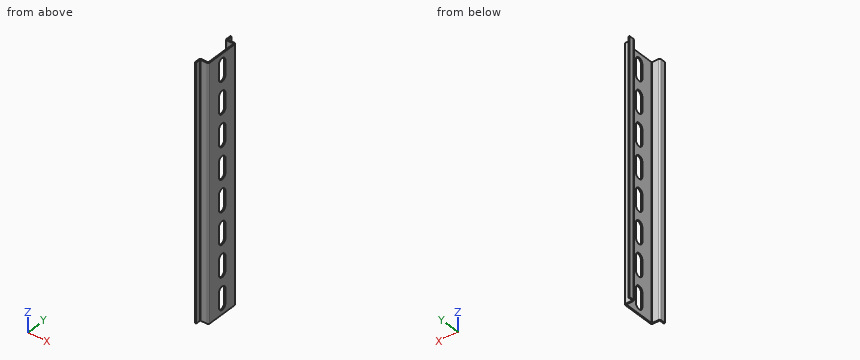
```python
from build123d import *

# Parameters (mm, degrees)
EXTRUDE_THIN1_DEPTH = 200.025
CUT_EXTRUDE1_START  = -8.5
CUT_EXTRUDE1_DEPTH  = 9.5
LPATTERN1_COUNT     = 32
LPATTERN1_PITCH     = 25
FILLET1_R           = 0.25
FILLET2_R           = 1.25


with BuildPart() as part:
    # Sketch3 → Extrude-Thin1 (new body)
    with BuildSketch(Plane.XY):
        Polygon((-6.5, 17.5), (-6.5, 13.5), (0, 13.5), (0, -13.5), (-6.5, -13.5), (-6.5, -17.5), (-7.5, -17.5), (-7.5, -12.5), (-1, -12.5), (-1, 12.5), (-7.5, 12.5), (-7.5, 17.5), align=None)
    extrude(amount=EXTRUDE_THIN1_DEPTH)

    # Sketch4 → Cut-Extrude1 (cut)
    with BuildSketch(Plane(origin=(0, 0, 0), x_dir=(0, 0, -1), z_dir=(1, 0, 0)).offset(CUT_EXTRUDE1_START)):
        with BuildLine():
            Line((-6.65, -3.15), (-18.35, -3.15))
            ThreePointArc((-18.35, -3.15), (-21.5, 0), (-18.35, 3.15))
            Line((-18.35, 3.15), (-6.65, 3.15))
            ThreePointArc((-6.65, 3.15), (-3.5, 0), (-6.65, -3.15))
        make_face()
    cut_extrude1 = extrude(amount=CUT_EXTRUDE1_DEPTH, mode=Mode.SUBTRACT)

    # LPattern1: Cut-Extrude1 ×32
    with Locations(*[(0, 0, i * LPATTERN1_PITCH) for i in range(1, LPATTERN1_COUNT)]):
        add(cut_extrude1, mode=Mode.SUBTRACT)

    # Fillet1
    fillet1_edges = [part.edges().sort_by_distance(p)[0] for p in [
        (-6.5, 13.5, 100.0125),
        (-6.5, -13.5, 100.0125),
        (-1, -12.5, 100.0125),
        (-1, 12.5, 100.0125),
    ]]
    fillet(fillet1_edges, radius=FILLET1_R)

    # Fillet2
    fillet2_edges = [part.edges().sort_by_distance(p)[0] for p in [
        (0, 13.5, 100.0125),
        (0, -13.5, 100.0125),
        (-7.5, -12.5, 100.0125),
        (-7.5, 12.5, 100.0125),
    ]]
    fillet(fillet2_edges, radius=FILLET2_R)


solid = part.part
```
Geometry check sheet. Reference: the model listing, model coordinates, mm. Round coordinates to 2 decimals unless told otherwise and drop trailing zeros. Order: outer loops, then holes, each group sorted by start corner. A loop starts at its lowest first (then second) coordinate and runs counter-clockwise, first axis right, second up. Notation, with made-up numbers: (58.5, -38.5) - (80.5, -38.5) arc R30 cw to (80.5, -5.5) - close; hole circle Ø7 at (-2, -31.5). An arc over 180 degrees is marked (long way). Use a Markdown table: item, result. Add a question column.
(1) Sectioned sample at D-D, the plane y = 1.5. Count the separate pieces of the cut face and the enclosed holes in it, and give its area (3 significant figures).
(2) Sectioned sample at B-B, the plane z = 125. Enter the section's corners in (x, y), and give its area (3 significant figures).
(3) Sectioned sample at C-C, the plane z = 15.5. Enter the section's corners in (x, y), and give its area (3 significant figures).
(4) Sectioned sample at A-A, the plane x = -4.25. Enter the section's corners in (y, z) (3 decimals), and give its area (3 significant figures).
(5) Depth check by flat-ended pin: pin 1 (1 mm diameter, centred on x = -3, y = 4, fed in from -Z); pin 2 (12 mm diameter, centred on y = -1, z = 104, fed in from -X); pin 3 (0.5 mm diameter, centred on x = -0.5, z = 188.5, fed in from -Y); pin 4 (1.1 mm diameter, centred on x = -0.5, z = 87.5, fed in from +Y). Enter the tip coordinate at first touch or a pass-through.
(6) Material ranges on line 1 along Y through (x, z) = (-3, 12.5); line 2 along X through (y, z) = (9, 89); line 3 along X through (y, z) = (15, 14.5), recorded low to high. Write a range as [from, to].
Answers below:
| question | item | result |
|---|---|---|
| 1 | separate pieces | 9 |
| 1 | enclosed holes | 0 |
| 1 | area | 62.1 mm² |
| 2 | outline | (-7.5, -17.5) - (-6.5, -17.5) - (-6.5, -13.75) arc R0.25 cw to (-6.25, -13.5) - (-1.25, -13.5) arc R1.25 ccw to (0, -12.25) - (0, 12.25) arc R1.25 ccw to (-1.25, 13.5) - (-6.25, 13.5) arc R0.25 cw to (-6.5, 13.75) - (-6.5, 17.5) - (-7.5, 17.5) - (-7.5, 13.75) arc R1.25 ccw to (-6.25, 12.5) - (-1.25, 12.5) arc R0.25 cw to (-1, 12.25) - (-1, -12.25) arc R0.25 cw to (-1.25, -12.5) - (-6.25, -12.5) arc R1.25 ccw to (-7.5, -13.75) - close |
| 2 | area | 46.7 mm² |
| 3 | outline | (-7.5, -17.5) - (-6.5, -17.5) - (-6.5, -13.75) arc R0.25 cw to (-6.25, -13.5) - (-1.25, -13.5) arc R1.25 ccw to (0, -12.25) - (0, -3.15) - (-1, -3.15) - (-1, -12.25) arc R0.25 cw to (-1.25, -12.5) - (-6.25, -12.5) arc R1.25 ccw to (-7.5, -13.75) - close; (-7.5, 13.75) arc R1.25 ccw to (-6.25, 12.5) - (-1.25, 12.5) arc R0.25 cw to (-1, 12.25) - (-1, 3.15) - (0, 3.15) - (0, 12.25) arc R1.25 ccw to (-1.25, 13.5) - (-6.25, 13.5) arc R0.25 cw to (-6.5, 13.75) - (-6.5, 17.5) - (-7.5, 17.5) - close |
| 3 | area | 40.4 mm² |
| 4 | outline | (-13.5, 0) - (-12.5, 0) - (-12.5, 200.025) - (-13.5, 200.025) - close; (12.5, 0) - (13.5, 0) - (13.5, 200.025) - (12.5, 200.025) - close |
| 4 | area | 400 mm² |
| 5 | pin 1 | through |
| 5 | pin 2 | x = -1 |
| 5 | pin 3 | y = -13.4 |
| 5 | pin 4 | y = 13.48 |
| 6 | line 1 | [-13.5, -12.5], [12.5, 13.5] |
| 6 | line 2 | [-1, 0] |
| 6 | line 3 | [-7.5, -6.5] |
